The listing builds one solid part. Answer for the finished solid, in the listing's coordinates (mm). Give positions to 0.01 mm unless a question says otherwise; leave off trailing zeros. Write each loop counter-clockwise with the first axis right and the second up, starting at its lowest first coordinate (ties: lowest second). Pieces come first, ordered by that corner, then holes.
```python
from build123d import *

# Parameters (mm, degrees)
BOSS_EXTRU_1_DEPTH         = 5
CONG_1_R                   = 3
ESQUISSE2_R                = 3
PER_AGE_PROFIL_DEPTH       = 6
ESQUISSE3_R                = 1.5
PER_AGE_ENCODEUR_DEPTH     = 6
POCHE_ROUE_ENCODEUSE_DEPTH = 6
CONG_2_R                   = 6
CONG_3_R                   = 3
ESQUISSE5_R                = 2.2
PER_AGE_BLOC_MOTEUR_DEPTH  = 6.0000001
ESQUISSE6_W                = 30
ESQUISSE6_H                = 66
POCHE_ROUE_MOTRICE_DEPTH   = 6.0000001
ESQUISSE7_R                = 3.5
PER_AGE_PATIN_DEPTH        = 6.0000001


with BuildPart() as part:
    # Esquisse1 → Boss.-Extru.1 (new body)
    with BuildSketch(Plane(origin=(0, 0, 0), x_dir=(1, 0, 0), z_dir=(0, 1, 0))):
        Polygon((-155, 125), (155, 125), (180, 100), (180, -100), (155, -125), (-155, -125), (-180, -100), (-180, 100), align=None)
    extrude(amount=BOSS_EXTRU_1_DEPTH)

    # Congé1
    cong_1_edges = [part.edges().sort_by_distance(p)[0] for p in [
        (180, 2.5, -100),
        (180, 2.5, 100),
        (155, 2.5, 125),
        (-155, 2.5, 125),
        (-180, 2.5, 100),
        (-180, 2.5, -100),
        (-155, 2.5, -125),
        (155, 2.5, -125),
    ]]
    fillet(cong_1_edges, radius=CONG_1_R)

    # Esquisse2 → Perçage Profilé (cut, through all)
    with BuildSketch(Plane(origin=(0, 5, 0), x_dir=(1, 0, 0), z_dir=(0, 1, 0))):
        with Locations((-157, -65)):
            Circle(ESQUISSE2_R)
        with Locations((-157, 65)):
            Circle(ESQUISSE2_R)
        with Locations((157, -65)):
            Circle(ESQUISSE2_R)
        with Locations((157, 65)):
            Circle(ESQUISSE2_R)
    extrude(amount=-PER_AGE_PROFIL_DEPTH, mode=Mode.SUBTRACT)

    # Esquisse3 → Perçage Encodeur (cut, through all)
    with BuildSketch(Plane(origin=(0, 5, 0), x_dir=(1, 0, 0), z_dir=(0, 1, 0))):
        with Locations((-153.5, 19.5)):
            Circle(ESQUISSE3_R)
        with Locations((-153.5, -19.5)):
            Circle(ESQUISSE3_R)
        with Locations((153.5, -19.5)):
            Circle(ESQUISSE3_R)
        with Locations((153.5, 19.5)):
            Circle(ESQUISSE3_R)
    extrude(amount=-PER_AGE_ENCODEUR_DEPTH, mode=Mode.SUBTRACT)

    # Esquisse4 → Poche Roue Encodeuse (cut, through all)
    with BuildSketch(Plane(origin=(0, 5, 0), x_dir=(1, 0, 0), z_dir=(0, 1, 0))):
        with BuildLine():
            Line((168.5, -15), (154.5, -15))
            ThreePointArc((154.5, -15), (153.792893219, -14.707106781), (153.5, -14))
            Line((153.5, -14), (153.5, 14))
            ThreePointArc((153.5, 14), (153.792893219, 14.707106781), (154.5, 15))
            Line((154.5, 15), (168.5, 15))
            Line((168.5, 15), (168.5, 32.5))
            Line((168.5, 32.5), (177, 32.5))
            Line((177, 32.5), (177, -32.5))
            Line((177, -32.5), (168.5, -32.5))
            Line((168.5, -32.5), (168.5, -15))
        make_face()
        with BuildLine():
            Line((-153.5, -14), (-153.5, 14))
            ThreePointArc((-153.5, 14), (-153.792893219, 14.707106781), (-154.5, 15))
            Line((-154.5, 15), (-168.5, 15))
            Line((-168.5, 15), (-168.5, 32.5))
            Line((-168.5, 32.5), (-177, 32.5))
            Line((-177, 32.5), (-177, -32.5))
            Line((-177, -32.5), (-168.5, -32.5))
            Line((-168.5, -32.5), (-168.5, -15))
            Line((-168.5, -15), (-154.5, -15))
            ThreePointArc((-154.5, -15), (-153.792893219, -14.707106781), (-153.5, -14))
        make_face()
    extrude(amount=-POCHE_ROUE_ENCODEUSE_DEPTH, mode=Mode.SUBTRACT)

    # Congé2
    cong_2_edges = [part.edges().sort_by_distance(p)[0] for p in [
        (-177, 2.5, 32.5),
        (-177, 2.5, -32.5),
        (177, 2.5, -32.5),
        (177, 2.5, 32.5),
    ]]
    fillet(cong_2_edges, radius=CONG_2_R)

    # Congé3
    cong_3_edges = [part.edges().sort_by_distance(p)[0] for p in [
        (168.5, 2.5, 32.5),
        (168.5, 2.5, -32.5),
        (-168.5, 2.5, 32.5),
        (-168.5, 2.5, -32.5),
    ]]
    fillet(cong_3_edges, radius=CONG_3_R)

    # Esquisse5 → Perçage Bloc Moteur (cut, through all)
    with BuildSketch(Plane(origin=(0, 5, 0), x_dir=(1, 0, 0), z_dir=(0, 1, 0))):
        with Locations((-113, 15)):
            Circle(ESQUISSE5_R)
        with Locations((-113, -15)):
            Circle(ESQUISSE5_R)
        with Locations((-50, -15)):
            Circle(ESQUISSE5_R)
        with Locations((-50, 15)):
            Circle(ESQUISSE5_R)
        with Locations((50, 15)):
            Circle(ESQUISSE5_R)
        with Locations((50, -15)):
            Circle(ESQUISSE5_R)
        with Locations((113, -15)):
            Circle(ESQUISSE5_R)
        with Locations((113, 15)):
            Circle(ESQUISSE5_R)
    extrude(amount=-PER_AGE_BLOC_MOTEUR_DEPTH, mode=Mode.SUBTRACT)

    # Esquisse6 → Poche Roue Motrice (cut, through all)
    with BuildSketch(Plane(origin=(0, 5, 0), x_dir=(1, 0, 0), z_dir=(0, 1, 0))):
        with Locations((-134, 0)):
            Rectangle(ESQUISSE6_W, ESQUISSE6_H)
        with Locations((134, 0)):
            Rectangle(ESQUISSE6_W, ESQUISSE6_H)
    extrude(amount=-POCHE_ROUE_MOTRICE_DEPTH, mode=Mode.SUBTRACT)

    # Esquisse7 → Perçage Patin (cut, through all)
    with BuildSketch(Plane(origin=(0, 5, 0), x_dir=(1, 0, 0), z_dir=(0, 1, 0))):
        with Locations((-155, 100)):
            Circle(ESQUISSE7_R)
        with Locations((-155, -100)):
            Circle(ESQUISSE7_R)
        with Locations((155, -100)):
            Circle(ESQUISSE7_R)
        with Locations((155, 100)):
            Circle(ESQUISSE7_R)
    extrude(amount=-PER_AGE_PATIN_DEPTH, mode=Mode.SUBTRACT)


solid = part.part
```
Item 1: A cutting plane is placed at B-B, the plane y = 2.6. Count the separate pieces of the cut face and the enclosed holes in it, plus the area to 3 significant figures.
Conclusion:
separate pieces: 1
enclosed holes: 24
area: 82,400 mm2
Item 2: Consider probe 1 along Z at (x, y) = (-50, 1.55); probe 2 along Z at (x, y) = (-138, 1.7); probe 3 along X at (y, z) = (1.2, 100). Determine where each line is inside the solid, lowest interval first.
Conclusion:
probe 1: z = -125 to -17.2, -12.8 to 12.8, 17.2 to 125
probe 2: z = -125 to -33, 33 to 125
probe 3: x = -179.73 to -158.5, -151.5 to 151.5, 158.5 to 179.73
Item 3: Determine the mould class of faces 1 (the face through (167, 2, -113)), 2 (the face through (158.233, 2.535, 101.341)), 3 (the face through (3, 0, -2)) for opening direction Z: pulls with the +Z half, pulls with the -Z half, needs draft (parallel to the pull), parting line crosses it, or undercut.
Conclusion:
face 1: pulls with the -Z half
face 2: undercut
face 3: needs draft
Item 4: Each of these flat-tipped pins is pushed along its axis until it touches: P1, Ø2.5, axis at x = 160.5, y = 2.5, coming from the -Z side; P2, Ø1.5, axis at x = -162.5, y = 1.5, coming from the -Z side. Where does it stop, or does it pass through?
Conclusion:
P1: stops at z = -120.75
P2: stops at z = -118.25
Item 5: A cutting plane is placed at A-A, the plane x = 130.5. Give the vertices of the cut face in (y, z), plus the area to 3 significant figures.
Conclusion:
outline: (0, -125) - (5, -125) - (5, -33) - (0, -33) - close; (0, 33) - (5, 33) - (5, 125) - (0, 125) - close
area: 920 mm2
